Autodesk Inventor part; units mm, degrees
ref_plane "YZ Plane" through (0, 0, 0) normal (1, 0, 0) x (0, 1, 0)
ref_plane "XZ Plane" through (0, 0, 0) normal (0, 1, 0) x (-1, 0, 0)
ref_plane "XY Plane" through (0, 0, 0) normal (0, 0, 1) x (1, 0, 0)
sketch "Sketch1" plane through (0, 0, 0) normal (0, 0, 1) x (1, 0, 0)
  circle A0 centre (0, 0) radius 40
  dimension "d0" = 80
extrude "Extrusion1" add sketch "Sketch1" along normal blind 100
sketch "Sketch2" plane through (0, 0, 100) normal (0, 0, 1) x (1, 0, 0)
  circle A0 centre (0, 0) radius 25.5
  dimension "d3" = 51
extrude "Extrusion2" add sketch "Sketch2" along normal blind 3
chamfer "Chamfer1" distance 0.6 angle 45 1 edges at (-25.5, 0, 103)
sketch "Sketch3" plane through (0, 0, 103) normal (0, 0, 1) x (1, 0, 0)
  circle A0 centre (0, 0) radius 21
  dimension "d9" = 42
extrude "SensorCutout" cut sketch "Sketch3" against normal blind 17.5
thread "Thread1"
sketch "Sketch4" plane through (0, 0, 85.5) normal (0, 0, 1) x (1, 0, 0)
  line L0 (-16, 11) -> (16, 11)
  line L1 (16, 11) -> (16, -11)
  line L2 (16, -11) -> (-16, -11)
  line L3 (-16, -11) -> (-16, 11)
  circle A0 centre (0, 0) radius 21
  point P0 (16, 0)
  point P1 (0, 11)
  dimension "d14" = 32
  dimension "d15" = 22
extrude "SensorFrame" add sketch "Sketch4" along normal blind 8.5
fillet "Fillet1" radius 2 4 edges at (-16, 11, 89.75) (-16, -11, 89.75) (16, 11, 89.75) (16, -11, 89.75)
chamfer "Chamfer2" distance 1 angle 45 4 edges at (0, 11, 94) (16, 0, 94) (0, -11, 94) (-16, 0, 94)
properties part number "RisingCam-IMX571"
The listing builds one solid part. Answer for the finished solid, in the listing's coordinates (mm). A direction names the side the tool comes from. Round coordinates to 2 decimals unless told otherwise and drop trailing zeros. Loops run counter-clockwise (first coordinate to the right, second up) from the corner with the lowest first, then second, coordinate; pieces in that order, holes last. Notation, with made-up numbers: (28, 88) - (40, 88) arc R26 ccw to (40, 126) - close; hole circle Ø1 at (84, 56). An arc over 180 degrees is marked (long way). Use one line per item in the form item = value. Start each with the question number.
1. A tool of negligible diameter and unlimited length cuts with its end or side. For faces 1 (the face through (-11.2, -18.3, 103)), 2 (the face through (0, -11, 89)), from which of +Z, -Z, +X, -X, +Y, -Y can it reach the whole face along a straight path? Write none if from no direction.
2. Given pin 1 Ø12.5 at (x, y) = (-5, 5) entering from +Z; pin 2 Ø1 at (y, z) = (-5.5, 29) entering from -X; pin 3 Ø12 at (x, z) = (1.5, 79.5) entering from -Y, each flat-ended and moving along its own axis, determine where each tip first touches the part or whether it passes through.
3. The part is cut by section B-B on y = 0. Determine the outline of the cut face in (x, z).
4. Consider line 1 (Y direction, x = 0, z = 99); line 2 (Y direction, x = 0, z = 101); line 3 (Z direction, x = 12.5, y = -7). Determine where each line is inside the solid, lowest interval first. Write a range as [from, to].
5. The part is cut by section D-D on x = 29. Determine the outline of the cut face in (y, z), then the cut area to 3 significant figures.
6. The part is cut by section A-A on x = 0. Determine the outline of the cut face in (y, z).
7. The part is cut by section C-C on z = 72. Determine the outline of the cut face in (x, y).
8. For a pull along X with two mould halves and no side action, classify faces 3 (the face through (-1, 1, 0)), 4 (the face through (-8.67, 39.05, 49.3)), 5 (the face through (15.68, -10.71, 93.4)) as pulls with the +X half, pulls with the -X half, needs draft (parallel to the pull), parting line crosses it, or undercut.
Geometry check:
q1.face_1 = +Z, +X, -X, +Y, -Y
q1.face_2 = +Z
q2.pin_1 = 93.25
q2.pin_2 = -39.69
q2.pin_3 = -40
q3.outline = (-40, 0) - (40, 0) - (40, 100) - (25.5, 100) - (25.5, 102.4) - (24.9, 103) - (21, 103) - (21, 94) - (17, 94) - (16, 93) - (16, 85.5) - (-16, 85.5) - (-16, 93) - (-17, 94) - (-21, 94) - (-21, 103) - (-24.9, 103) - (-25.5, 102.4) - (-25.5, 100) - (-40, 100) - close
q4.line_1 = [-40, -21], [21, 40]
q4.line_2 = [-25.5, -21], [21, 25.5]
q4.line_3 = [0, 85.5]
q5.outline = (-27.55, 0) - (27.55, 0) - (27.55, 100) - (-27.55, 100) - close
q5.area = 5,510 mm^2
q6.outline = (-40, 0) - (40, 0) - (40, 100) - (25.5, 100) - (25.5, 102.4) - (24.9, 103) - (21, 103) - (21, 94) - (12, 94) - (11, 93) - (11, 85.5) - (-11, 85.5) - (-11, 93) - (-12, 94) - (-21, 94) - (-21, 103) - (-24.9, 103) - (-25.5, 102.4) - (-25.5, 100) - (-40, 100) - close
q7.outline = circle Ø80 at (0, 0)
q8.face_3 = needs draft
q8.face_4 = parting line crosses it
q8.face_5 = undercut
